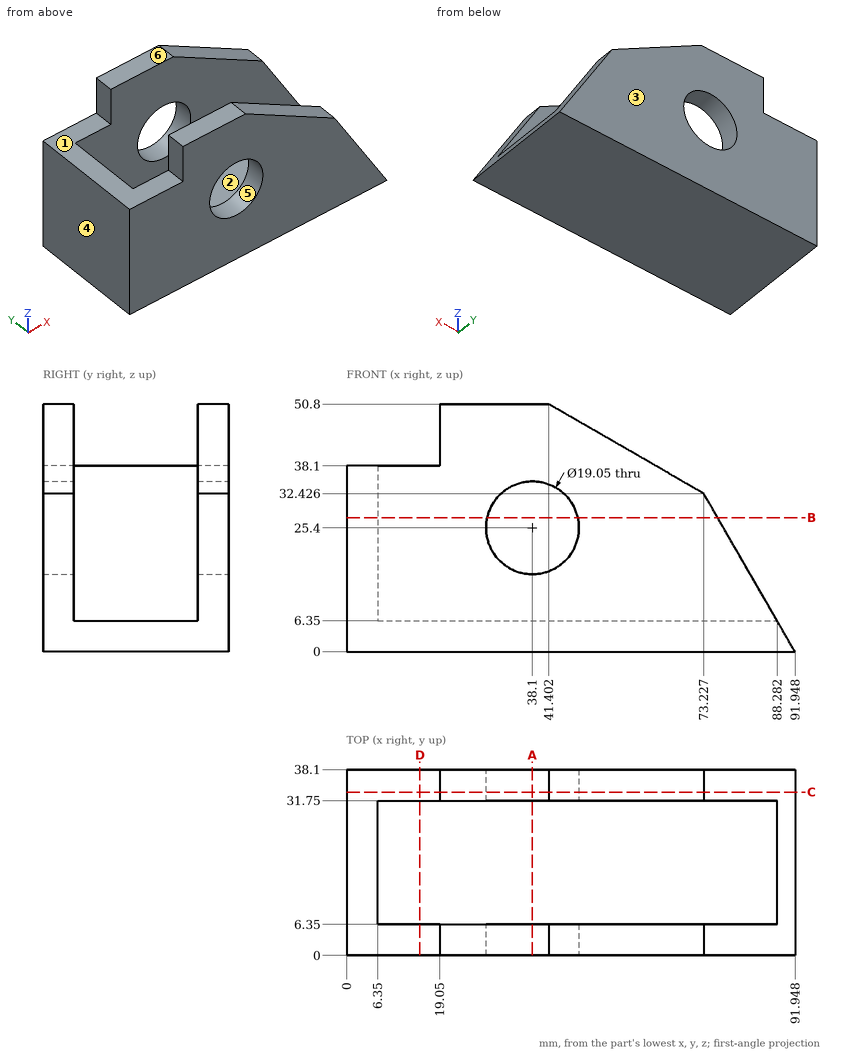
Geometry: see drawing. Coordinates: mm, zero at the bounding-box minimum. A direction names the side the tool comes from. Round coordinates to 2 decimals unless told otherwise and drop trailing zeros. Loops run counter-clockwise (first coordinate to the right, second up) from the corner with the lowest first, then second, coordinate; pieces in that order, holes last. Notation, with made-up numbers: (13, -13) -> (46, -13) arc R24 ccw to (46, 2) -> close; hole circle Ø3 at (55.25, -23). An arc over 180 degrees is marked (long way). One line per question, with ' | ' between items. Start each with the question number.
1. Set-up query: the marked faces 1, 2 and 3. Return all of +Z, -Z, +X, -X, +Y, -Y with unobstructed straight access to the full face (end or side cutting, diameter ignored); none if empty.
2. Contact query for flat-ended pins moving along their axis: pin 1 (1.5 mm diameter, centred on x = 55, y = 33.5, fed in from +Z); pin 2 (4 mm diameter, centred on x = 62.5, z = 25, fed in from -Y); pin 3 (15 mm diameter, centred on x = 12.5, y = 16.5, fed in from +Z); pin 4 (5 mm diameter, centred on y = 3, z = 44, fed in from -X). Output: stop coordinate, or through.
3. Section C-C on y = 33.5. Output: boundary loops of the cut face in (x, z) (3 decimals), and give its area (3 significant figures).
4. Mould query, pull axis X, two halves, no side actions, for the marked faces 4, 5 and 6. Classes: pulls with the +X half, pulls with the -X half, needs draft (parallel to the pull), parting line crosses it, or undercut.
5. Section A-A on x = 38.1. Output: boundary loops of the cut face in (y, z) (3 decimals).
6. Section D-D on x = 15. Output: boundary loops of the cut face in (y, z), and give its area (3 significant figures).
7. Section B-B on z = 27.5. Output: boundary loops of the cut face in (x, y).
8. Line query: line 1 along Z through (x, y) = (38, 2); line 2 along Y through (x, z) = (53, 19.5); line 3 along Z through (x, y) = (7, 3). Output: solid intervals per line, ascending. Write a range as [from, to].
Returned:
1) face 1: +Z, -X, +Y, -Y | face 2: +Z, +X | face 3: +Z, -Z, +X, -X, +Y
2) pin 1: stops at z = 43.38 | pin 2: stops at y = 0 | pin 3: stops at z = 38.1 | pin 4: stops at x = 19.05
3) outline: (0, 0) -> (91.948, 0) -> (73.227, 32.426) -> (41.402, 50.8) -> (19.05, 50.8) -> (19.05, 38.1) -> (0, 38.1) -> close; hole circle Ø19.05 at (38.1, 25.4) | area: 3,200 mm2
4) face 4: pulls with the -X half | face 5: undercut | face 6: needs draft
5) outline: (0, 0) -> (38.1, 0) -> (38.1, 15.875) -> (31.75, 15.875) -> (31.75, 6.35) -> (6.35, 6.35) -> (6.35, 15.875) -> (0, 15.875) -> close; (0, 34.925) -> (6.35, 34.925) -> (6.35, 50.8) -> (0, 50.8) -> close; (31.75, 34.925) -> (38.1, 34.925) -> (38.1, 50.8) -> (31.75, 50.8) -> close
6) outline: (0, 0) -> (38.1, 0) -> (38.1, 38.1) -> (31.75, 38.1) -> (31.75, 6.35) -> (6.35, 6.35) -> (6.35, 38.1) -> (0, 38.1) -> close | area: 645 mm2
7) outline: (0, 0) -> (28.81, 0) -> (28.81, 6.35) -> (6.35, 6.35) -> (6.35, 31.75) -> (28.81, 31.75) -> (28.81, 38.1) -> (0, 38.1) -> close; (47.39, 0) -> (76.07, 0) -> (76.07, 6.35) -> (47.39, 6.35) -> close; (47.39, 31.75) -> (76.07, 31.75) -> (76.07, 38.1) -> (47.39, 38.1) -> close
8) line 1: z = [0, 15.88], [34.92, 50.8] | line 2: y = [0, 6.35], [31.75, 38.1] | line 3: z = [0, 38.1]
